Autodesk Inventor part; units mm, degrees
ref_plane "YZ Plane" through (0, 0, 0) normal (1, 0, 0) x (0, 1, 0)
ref_plane "XZ Plane" through (0, 0, 0) normal (0, 1, 0) x (-1, 0, 0)
ref_plane "XY Plane" through (0, 0, 0) normal (0, 0, 1) x (1, 0, 0)
sketch "Эскиз3" plane through (0, 0, 0) normal (0, 0, 1) x (1, 0, 0)
  line L0 (0, 0) -> (20, 0)
  line L1 (20, 0) -> (20, 25)
  line L2 (16, 29) -> (4, 29)
  line L3 (0, 25) -> (0, 0)
  line L4 (4, 29) -> (0, 25)
  line L5 (16, 29) -> (20, 25)
  point P0 (20, 29)
  point P1 (0, 29)
  dimension "d18" = 20
  dimension "d19" = 29
  dimension "d20" = 4
  dimension "d21" = 4
  dimension "d22" = 4
  dimension "d23" = 4
revolve "Вращение2" add sketch "Эскиз3" angle 360 about axis through (0, 0, 0) along (1, 0, 0)
sketch "Эскиз4" plane through (20, 0, 0) normal (1, 0, 0) x (0, 0, -1)
  point P0 (0, 0)
  point P1 (0, 0)
hole "Отверстие2" at (20, 0, 0) direction (-1, 0, 0) diameter 14 depth 6 tip angle 150 countersink diameter 16 countersink angle 90
thread "Резьба3"
properties part number "711131"
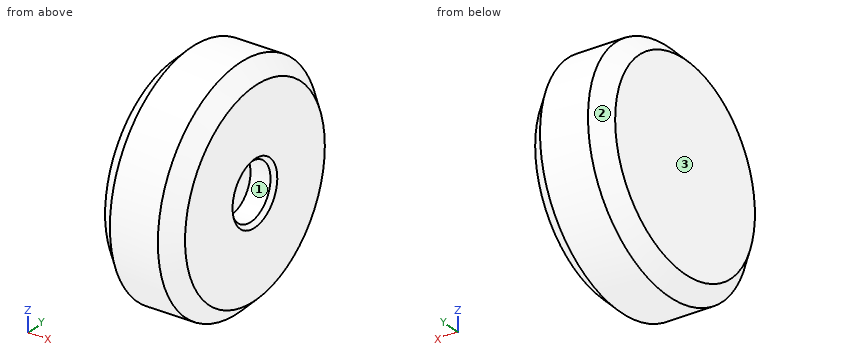
Can you work these out from the model? Positions are in its coordinate system, mm. Face numbers are marked on the shaded views. Coordinates: 2 decimals unless noted, no trailing zeros. Write each loop counter-clockwise with the first axis right and the second up, starting at its lowest first coordinate (ties: lowest second). Pieces come first, ordered by that corner, then holes. Notation, with made-up numbers: (-36.75, 43.5) - (-14.75, 43.5) arc R11 cw to (-14.75, 62.5) - close; hole circle Ø11 at (-33.75, 89.5). An arc over 180 degrees is marked (long way). Return JSON: item names as keys, results as strings. Group by question number.
Item 1: If we section it at B-B (x = 7): Write out the boundary of the cut face in (y, z).
Item 2: We'd pull the mould along Y, two halves only. Please class the marked faces 1, 2 and 3: pulls with the +Y half, pulls with the -Y half, needs draft (parallel to the pull), parting line crosses it, or undercut.
Item 3: I'm going to push flat-ended pins straight in: pin 1 Ø10 at (x, y) = (13.5, -21) entering from +Z; pin 2 Ø2 at (x, y) = (5.5, -6) entering from -Z; pin 3 Ø10 at (x, z) = (10.5, 13) entering from -Y. Where does each tip first touch, or does it pass through?
Item 4: If we section it at A-A (x = 3): Write out the boundary of the cut face in (y, z).
Item 5: Please list where these lines run through material, in increasing order: probe 1 along Z at (x, y) = (15.8, 0); probe 2 along Z at (x, y) = (17.7, 0); probe 3 along Y at (x, z) = (17.4, 0).
Return value:
{
 "1": {"outline": "circle Ø58 at (0, 0)"},
 "2": {"face 1": "undercut", "face 2": "parting line crosses it", "face 3": "needs draft"},
 "3": {"pin 1": "stops at z = 24.19", "pin 2": "stops at z = -28.57", "pin 3": "stops at y = -27.87"},
 "4": {"outline": "circle Ø56 at (0, 0)"},
 "5": {"probe 1": "z = -29 to -7, 7 to 29", "probe 2": "z = -27.3 to -7, 7 to 27.3", "probe 3": "y = -27.6 to -7, 7 to 27.6"}
}
